For this review, take the finished solid that the model builds, in its own axes (mm). A direction names the side the tool comes from. Round coordinates to 2 decimals unless told otherwise and drop trailing zeros. Write each loop counter-clockwise with the first axis right and the second up, starting at its lowest first coordinate (ties: lowest second). Pieces come first, ordered by that corner, then holes.
from build123d import *

# Parameters (mm, degrees)
SKETCH_R          = 48.1711
SKETCH_R_2        = 44.9961
PAD_DEPTH         = 12.7
SKETCH001_R       = 46.1645
SKETCH001_R_2     = 42.9895
PAD001_DEPTH      = 12.7
SKETCH002_R       = 2.0193
POCKET_DEPTH      = 76.2
POCKET_DEPTH_BACK = 76.2
SKETCH003_R       = 45.974
SKETCH003_R_2     = 36.6395
PAD002_DEPTH      = 2.54
SKETCH004_R       = 1.905
POCKET001_DEPTH   = 5.08
FILLET_R          = 0.635
FILLET001_R       = 1.778
FILLET002_R       = 0.635


with BuildPart() as part:
    # Sketch → Pad (new body)
    with BuildSketch(Plane.XY):
        Circle(SKETCH_R)
        Circle(SKETCH_R_2, mode=Mode.SUBTRACT)
    extrude(amount=PAD_DEPTH)

    # Sketch001 (on Face4 of Pad) → Pad001 (join)
    with BuildSketch(Plane.XY.offset(12.7)):
        Circle(SKETCH001_R)
        Circle(SKETCH001_R_2, mode=Mode.SUBTRACT)
    extrude(amount=PAD001_DEPTH)

    # Sketch002 → Pocket (cut, two sides)
    with BuildSketch(Plane.XZ) as pocket_sk:
        with Locations((0, 6.35)):
            Circle(SKETCH002_R)
    extrude(amount=POCKET_DEPTH, mode=Mode.SUBTRACT)
    extrude(pocket_sk.sketch, amount=-POCKET_DEPTH_BACK, mode=Mode.SUBTRACT)

    # Sketch003 → Pad002 (join)
    with BuildSketch(Plane.XY.offset(25.4)):
        Circle(SKETCH003_R)
        Circle(SKETCH003_R_2, mode=Mode.SUBTRACT)
    extrude(amount=-PAD002_DEPTH)

    # Sketch004 (on Face12 of Pad002) → Pocket001 (cut)
    with BuildSketch(Plane(origin=(0, 0, 22.86), x_dir=(1, 0, 0), z_dir=(0, 0, -1))):
        with Locations((0, 39.624)):
            Circle(SKETCH004_R)
        with Locations((0, -39.624)):
            Circle(SKETCH004_R)
    extrude(amount=-POCKET001_DEPTH, mode=Mode.SUBTRACT)

    # Fillet
    fillet_edges = [part.edges().sort_by_distance(p)[0] for p in [
        (-48.1711, 0, 0),
        (-44.9961, 0, 0),
    ]]
    fillet(fillet_edges, radius=FILLET_R)

    # Fillet001
    fillet001_edges = [part.edges().sort_by_distance(p)[0] for p in [
        (-46.1645, 0, 12.7),
    ]]
    fillet(fillet001_edges, radius=FILLET001_R)

    # Fillet002
    fillet002_edges = [part.edges().sort_by_distance(p)[0] for p in [
        (-46.1645, 0, 25.4),
    ]]
    fillet(fillet002_edges, radius=FILLET002_R)


solid = part.part
(1) For line 1 along Y through (x, z) = (0, 24.4); line 2 along Y through (x, z) = (2.5, 21.5); line 3 along Y through (x, z) = (0, 3.5), list the stretches that pass through material, from the lowest coordinate up.
Geometry check:
line 1: y = -46.16 to -41.53, -37.72 to -36.64, 36.64 to 37.72, 41.53 to 46.16
line 2: y = -46.1 to -42.92, 42.92 to 46.1
line 3: y = -48.17 to -45, 45 to 48.17
(2) We need section B-B, the plane x = 0. State how many separate pieces and enclosed holes the cut face has, and give its area (3 significant figures).
Geometry check:
separate pieces: 6
enclosed holes: 0
area: 149 mm2
(3) For pin 1 Ø8 at (x, z) = (-12.5, 18) entering from +Y; pin 2 Ø5.5 at (x, z) = (0, 6.35) entering from -Y; pin 3 Ø3.5 at (x, z) = (0, 6.35) entering from +Y; pin 4 Ø12 at (y, z) = (12.5, 22.5) entering from +X, all flat-tipped, find the tip position at first contact; note any pin that passes through.
Geometry check:
pin 1: stops at y = 45.38
pin 2: stops at y = -48.17
pin 3: passes through
pin 4: stops at x = 45.7
(4) We need section C-C, the plane z = 10.5. Give the boundary of the cut face in (x, y).
Geometry check:
outline: circle Ø96.34 at (0, 0); hole circle Ø89.99 at (0, 0)
(5) We need section A-A, the plane z = 21. Give the boundary of the cut face in (x, y), and give its area (3 significant figures).
Geometry check:
outline: circle Ø92.33 at (0, 0); hole circle Ø85.98 at (0, 0)
area: 889 mm2
(6) For faces 1 (the face through (44.03, 13.87, 19.55)), 2 (the face through (24.19, 37.94, 6.58)), 3 (the face through (-0.44, 46.54, 4.38)), list the 3-axis set-ups (+Z, -Z, +X, -X, +Y, -Y) from which the entire face can be reached by the end or side of a thin tool; tool diameter is ignored.
Geometry check:
face 1: +Z
face 2: -Z
face 3: +Y, -Y
(7) Mouldability with a two-part tool opening along X and no side actions: class faces 4 (the face through (-0.413, -37.764, 24.112)), 5 (the face through (0, -37, 25.4)), 6 (the face through (-10.443, -47.026, 6.583)), 7 (the face through (-9.319, -41.967, 17.709)) as pulls with the +X half, pulls with the -X half, needs draft (parallel to the pull), parting line crosses it, or undercut.
Geometry check:
face 4: undercut
face 5: needs draft
face 6: parting line crosses it
face 7: undercut
